Autodesk Inventor part; units mm, degrees
ref_plane "YZ Plane" through (0, 0, 0) normal (1, 0, 0) x (0, 1, 0)
ref_plane "XZ Plane" through (0, 0, 0) normal (0, 1, 0) x (-1, 0, 0)
ref_plane "XY Plane" through (0, 0, 0) normal (0, 0, 1) x (1, 0, 0)
sketch "Sketch1" plane through (0, 0, 0) normal (0, 0, 1) x (1, 0, 0)
  circle A0 centre (0, 0) radius 5.95
  dimension "d1" = 11.9
extrude "Extrusion1" add sketch "Sketch1" along normal mid plane 236.69
chamfer "Chamfer3" distance 0.5 angle 45 1 edges at (-5.95, 0, -118.345)
sketch "Sketch4" plane through (0, 0, 118.345) normal (0, 0, 1) x (1, 0, 0)
  circle A0 centre (0, 0) radius 6
extrude "Extrusion5" add sketch "Sketch4" along normal blind 3
properties part number "Plate Support" material "Aluminum 6061"
The model under review builds one solid part; all positions refer to its coordinate system, in mm. Round coordinates to 2 decimals unless told otherwise and drop trailing zeros. Loops run counter-clockwise (first coordinate to the right, second up) from the corner with the lowest first, then second, coordinate; pieces in that order, holes last. Notation, with made-up numbers: (72.5, 87.25) - (110.5, 87.25) arc R22 ccw to (110.5, 114.25) - close; hole circle Ø11 at (55.5, 67). An arc over 180 degrees is marked (long way). Use a Markdown table: item, result. Add a question column.
Q1. Insertion check: pin 1 Ø1 at (y, z) = (3.5, 55) entering from -X; pin 2 Ø4 at (x, z) = (4.5, -34.5) entering from +Y; pin 3 Ø4 at (y, z) = (2.5, 64.5) entering from +X. Each pin has a flat end and moves straight along its axis. Give the tip position at first contact, or say it passes through.
Q2. Add section A-A (z = -88.5). State the section outline as (x, y) points, plus the area to 3 significant figures.
Q3. For probe 1 along Y at (x, z) = (0, 75.5); probe 2 along X at (y, z) = (-0.75, 81); probe 3 along X at (y, z) = (-2.75, 56.5), list the stretches that pass through material, from the lowest coordinate up.
Worked answers:
| question | item | result |
|---|---|---|
| 1 | pin 1 | x = -5.14 |
| 1 | pin 2 | y = 5.4 |
| 1 | pin 3 | x = 5.93 |
| 2 | outline | circle Ø11.9 at (0, 0) |
| 2 | area | 111 mm² |
| 3 | probe 1 | -5.95 to 5.95 |
| 3 | probe 2 | -5.9 to 5.9 |
| 3 | probe 3 | -5.28 to 5.28 |
